```python
from build123d import *

# Parameters (mm, degrees)
SKETCH1_W                                    = 9
SKETCH1_H                                    = 5.5
BOSS_EXTRUDE1_DEPTH                          = 274
CUT_EXTRUDE2_DEPTH                           = 275
CBORE_FOR_SOCKET_HEAD_CAP_SCREW1_D           = 3.5
CBORE_FOR_SOCKET_HEAD_CAP_SCREW1_CBORE_D     = 6
CBORE_FOR_SOCKET_HEAD_CAP_SCREW1_CBORE_DEPTH = 3.5
LPATTERN1_COUNT                              = 14
LPATTERN1_PITCH                              = 20
CHAMFER1_SIZE                                = 0.2
CHAMFER2_SIZE                                = 0.3


with BuildPart() as part:
    # Sketch1 → Boss-Extrude1 (new body)
    with BuildSketch(Plane(origin=(-7, 0, 0), x_dir=(0, 0, -1), z_dir=(1, 0, 0))):
        with Locations((0, 2.75)):
            Rectangle(SKETCH1_W, SKETCH1_H)
    extrude(amount=BOSS_EXTRUDE1_DEPTH)

    # Sketch3 → Cut-Extrude2 (cut, through all)
    with BuildSketch(Plane(origin=(-7, 0, 0), x_dir=(0, 0, -1), z_dir=(1, 0, 0))):
        with BuildLine():
            Line((4.5, 5.04428602), (4.22, 4.882627944))
            ThreePointArc((4.22, 4.882627944), (3.942636741, 4.654893122), (3.753338798, 4.35))
            Line((3.753338798, 4.35), (3.1, 4.35))
            Line((3.1, 4.35), (3.1, 3.65))
            Line((3.1, 3.65), (3.753338798, 3.65))
            ThreePointArc((3.753338798, 3.65), (3.942636741, 3.345106878), (4.22, 3.117372056))
            Line((4.22, 3.117372056), (4.5, 2.95571398))
            Line((4.5, 2.95571398), (4.5, 5.04428602))
        make_face()
        with BuildLine():
            Line((-4.5, 5.04428602), (-4.5, 2.95571398))
            Line((-4.5, 2.95571398), (-4.22, 3.117372056))
            ThreePointArc((-4.22, 3.117372056), (-3.942636741, 3.345106878), (-3.753338798, 3.65))
            Line((-3.753338798, 3.65), (-3.1, 3.65))
            Line((-3.1, 3.65), (-3.1, 4.35))
            Line((-3.1, 4.35), (-3.753338798, 4.35))
            ThreePointArc((-3.753338798, 4.35), (-3.942636741, 4.654893122), (-4.22, 4.882627944))
            Line((-4.22, 4.882627944), (-4.5, 5.04428602))
        make_face()
    extrude(amount=CUT_EXTRUDE2_DEPTH, mode=Mode.SUBTRACT)

    # CBORE for Socket Head Cap Screw1 (through all)
    with Locations(Plane(origin=(0, 5.5, 0), x_dir=(1, 0, 0), z_dir=(0, 1, 0))):
        with Locations((0, 0)):
            cbore_for_socket_head_cap_screw1 = CounterBoreHole(CBORE_FOR_SOCKET_HEAD_CAP_SCREW1_D / 2, CBORE_FOR_SOCKET_HEAD_CAP_SCREW1_CBORE_D / 2, CBORE_FOR_SOCKET_HEAD_CAP_SCREW1_CBORE_DEPTH)

    # LPattern1: CBORE for Socket Head Cap Screw1 ×14
    with Locations(*[(i * LPATTERN1_PITCH, 0, 0) for i in range(1, LPATTERN1_COUNT)]):
        add(cbore_for_socket_head_cap_screw1, mode=Mode.SUBTRACT)

    # Chamfer1
    chamfer1_edges = [part.edges().sort_by_distance(p)[0] for p in [
        (130, 5.5, 4.5),
        (130, 5.5, -4.5),
    ]]
    chamfer(chamfer1_edges, length=CHAMFER1_SIZE)

    # Chamfer2
    chamfer2_edges = [part.edges().sort_by_distance(p)[0] for p in [
        (130, 0, -4.5),
        (130, 0, 4.5),
    ]]
    chamfer(chamfer2_edges, length=CHAMFER2_SIZE)


solid = part.part
```
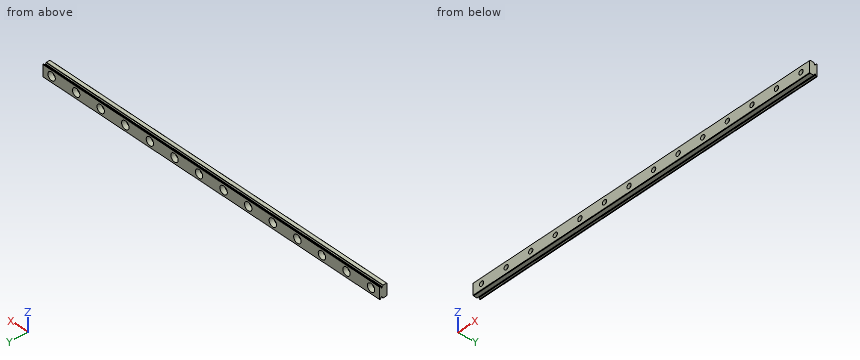
Model file for the job. Use its own axes, mm. Coordinates: 2 decimals unless noted, no trailing zeros. Loops run counter-clockwise (first coordinate to the right, second up) from the corner with the lowest first, then second, coordinate; pieces in that order, holes last. Notation, with made-up numbers: (82.5, 6) - (121.5, 6) arc R18 ccw to (121.5, 17) - close; hole circle Ø1 at (-20, -28.5). An arc over 180 degrees is marked (long way). Answer as a JSON object with one key per item and string values. Group by question number.
(1) Cut at A-A (y = 1.15). State how many separate pieces and enclosed holes the cut face has, then the cut area to 3 significant figures.
(2) Probe line 1 along Y through (x, z) = (236, -3.5); line 2 along Y through (x, z) = (167.5, 4.25); line 3 along Y through (x, z) = (42, 2). List the from-to ranges inside material, lowest first.
(3) Cut at C-C (x = 114). Give the cut face in (y, z), then the cut area to 3 significant figures.
(4) Flat gauge pins, fed straight in: pin 1 (3 mm diameter, centred on x = 198.5, z = -0.5, fed in from +Y); pin 2 (4.5 mm diameter, centred on x = 60, z = 0, fed in from +Y); pin 3 (0.8 mm diameter, centred on x = 186.5, y = 4, fed in from -Z). Where does each tip first touch, or does it go through?
Geometry says:
{
 "1": {"separate pieces": "1", "enclosed holes": "14", "area": "2,330 mm^2"},
 "2": {"line 1": "y = 0 to 3.65, 4.35 to 5.5", "line 2": "y = 0.05 to 3.1, 4.9 to 5.5", "line 3": "y = 0 to 2"},
 "3": {"outline": "(0, -4.2) - (0.3, -4.5) - (2.96, -4.5) - (3.12, -4.22) arc R1.1 cw to (3.65, -3.75) - (3.65, -3.1) - (4.35, -3.1) - (4.35, -3.75) arc R1.1 cw to (4.88, -4.22) - (5.04, -4.5) - (5.3, -4.5) - (5.5, -4.3) - (5.5, 4.3) - (5.3, 4.5) - (5.04, 4.5) - (4.88, 4.22) arc R1.1 cw to (4.35, 3.75) - (4.35, 3.1) - (3.65, 3.1) - (3.65, 3.75) arc R1.1 cw to (3.12, 4.22) - (2.96, 4.5) - (0.3, 4.5) - (0, 4.2) - close", "area": "46.1 mm^2"},
 "4": {"pin 1": "stops at y = 5.5", "pin 2": "stops at y = 2", "pin 3": "stops at z = -3.78"}
}
